Verification items for this drawing (mm, ordinates from the low corner). A direction names the side the tool comes from. Coordinates: 2 decimals unless noted, no trailing zeros. Order: outer loops, then holes, each group sorted by start corner. A loop starts at its lowest first (then second) coordinate and runs counter-clockwise, first axis right, second up. Notation, with made-up numbers: (35.5, 7) -> (57.5, 7) arc R16 ccw to (57.5, 14) -> close; hole circle Ø3 at (45, -12). An arc over 180 degrees is marked (long way). Write each question's results on one line, items separated by ' | '. Start each with the question number.
(1) Thickness scan on probe 1 along Z at (x, y) = (42, 25); probe 2 along Z at (x, y) = (32, 25); probe 3 along Y at (x, z) = (27, 27). Record the ranges inside material, lowest first. Write a range as [from, to].
(2) Cross-section at C-C on y = 11. Enter the section's corners in (x, z).
(3) Draft check along Y on the marked faces 1, 2 and 3. Enter one of: +Y half, -Y half, draft (parallel to the pull), parting line (faces both ways), or undercut.
(4) Go/stop test with flat-tipped pins: pin 1 (6.5 mm diameter, centred on y = 29, z = 19.5, fed in from -X); pin 2 (2 mm diameter, centred on x = 24, z = 24.5, fed in from -Y); pin 3 (1 mm diameter, centred on x = 37, z = 32.5, fed in from +Y). Record where each tip stops, or that it passes through.
(5) Set-up check for the marked faces 4, 5 and 6: record each of +Z, -Z, +X, -X, +Y, -Y from which the full face is reachable in a straight line by a thin tool's end or side.
(6) Cross-section at A-A on x = 40. Enter the section's corners in (y, z), and give its area (3 significant figures).
(7) Cross-section at B-B on z = 40. Enter the section's corners in (x, y) (3 decimals).
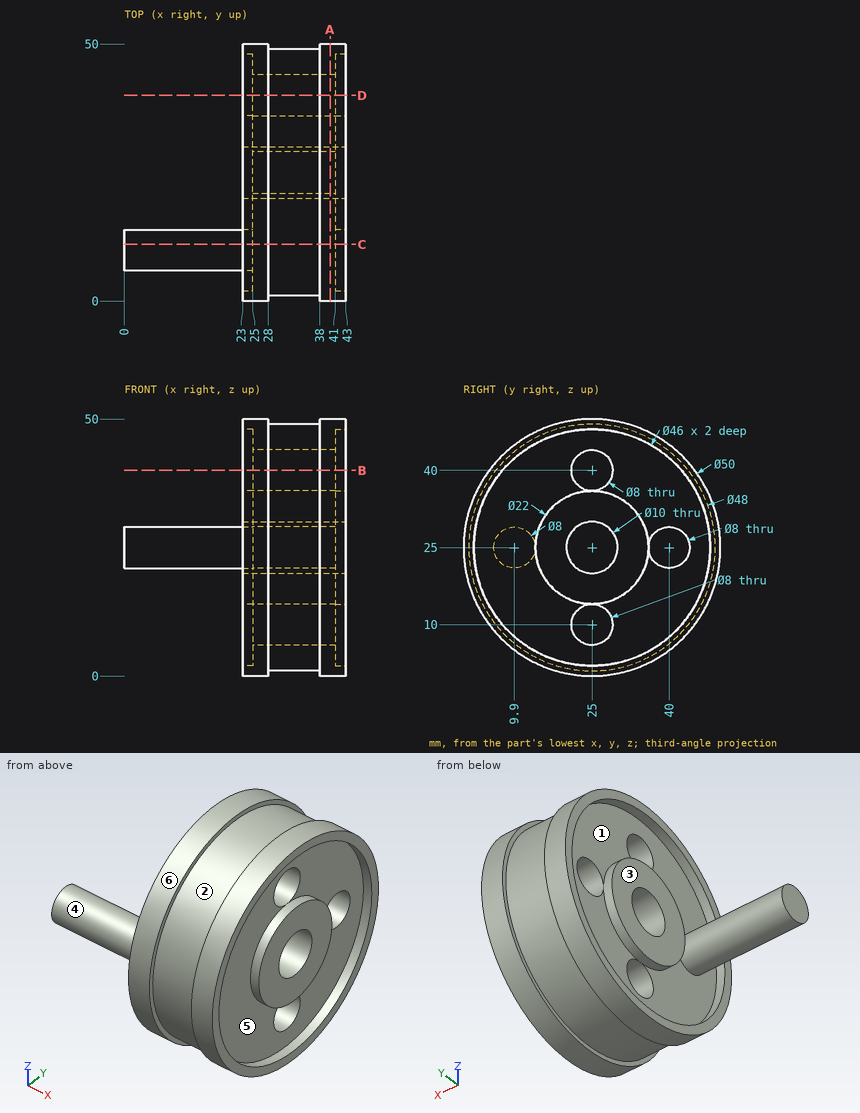
Results are:
1) probe 1: z = [0, 2], [14, 20], [30, 36], [48, 50] | probe 2: z = [1, 6], [14, 20], [30, 36], [44, 49] | probe 3: y = [0.08, 20.42], [29.58, 36.54], [43.46, 49.92]
2) outline: (0, 21.15) -> (25, 21.15) -> (25, 6.75) -> (23, 6.75) -> (23, 4.29) -> (28, 4.29) -> (28, 5.51) -> (38, 5.51) -> (38, 4.29) -> (43, 4.29) -> (43, 6.75) -> (41, 6.75) -> (41, 43.25) -> (43, 43.25) -> (43, 45.71) -> (38, 45.71) -> (38, 44.49) -> (28, 44.49) -> (28, 45.71) -> (23, 45.71) -> (23, 43.25) -> (25, 43.25) -> (25, 28.85) -> (0, 28.85) -> close
3) face 1: undercut | face 2: parting line | face 3: draft
4) pin 1: stops at x = 23 | pin 2: stops at y = 0 | pin 3: stops at y = 47.96
5) face 4: -X | face 5: +X | face 6: +X, -X
6) outline: circle Ø50 at (25, 25); hole circle Ø10 at (25, 25); hole circle Ø8 at (25, 10); hole circle Ø8 at (25, 40); hole circle Ø8 at (40, 25) | area: 1,730 mm2
7) outline: (23, 5) -> (28, 5) -> (28, 6.265) -> (38, 6.265) -> (38, 5) -> (43, 5) -> (43, 7.564) -> (41, 7.564) -> (41, 21) -> (25, 21) -> (25, 7.564) -> (23, 7.564) -> close; (23, 42.436) -> (25, 42.436) -> (25, 29) -> (41, 29) -> (41, 42.436) -> (43, 42.436) -> (43, 45) -> (38, 45) -> (38, 43.735) -> (28, 43.735) -> (28, 45) -> (23, 45) -> close
